CAD build for the part. Positions are in the model's coordinates, mm. Face numbers are marked on the shaded views. A direction names the side the tool comes from. Coordinates: 2 decimals unless noted, no trailing zeros. One line per item, written item: value.
from build123d import *

# Parameters (mm, degrees)
ESBO_O1_R           = 19
ESBO_O1_R_2         = 15
CONTRA_CENTRO_DEPTH = 12
CHANFRO1_SIZE       = 3.5
CHANFRO1_SIZE2      = 2


with BuildPart() as part:
    # Esboço1 → CONTRA CENTRO (new body)
    with BuildSketch(Plane.XY):
        Circle(ESBO_O1_R)
        Circle(ESBO_O1_R_2, mode=Mode.SUBTRACT)
    extrude(amount=CONTRA_CENTRO_DEPTH)

    # Chanfro1
    chanfro1_edges = [part.edges().sort_by_distance(p)[0] for p in [
        (-19, 0, 0),
    ]]
    chanfro1_side = [part.faces().sort_by_distance(p)[0] for p in [
        (-18.462598846, 0, 0),
    ]]
    chamfer(chanfro1_edges, length=CHANFRO1_SIZE, length2=CHANFRO1_SIZE2, reference=chanfro1_side[0])

    # Esboço2 → AA26234 (revolve)
    with BuildSketch(Plane(origin=(0, 0, 0), x_dir=(0, 0, -1), z_dir=(1, 0, 0)), mode=Mode.PRIVATE) as aa26234_sk:
        Polygon((-2.5, 19), (-10, 19), (-10, 24.5), (-12, 27.437165192), (-11.173430596, 28), (-9, 24.808137652), (-9, 20), (-7.5, 20), (-7.5, 23.763932023), (-9.894427191, 28.552786405), (-9, 29), (-6.5, 24), (-6.5, 20), (-5.5, 20), (-5.5, 23.763932023), (-7.894427191, 28.552786405), (-7, 29), (-4.5, 24), (-4.5, 20), (-3.5, 20), (-3.5, 23.763932023), (-5.894427191, 28.552786405), (-5, 29), (-2.5, 24), align=None)
    revolve(aa26234_sk.sketch.rotate(Axis((0, 0, 10), (0, 0, -1)), 90), axis=Axis((0, 0, 10), (0, 0, -1)))


solid = part.part
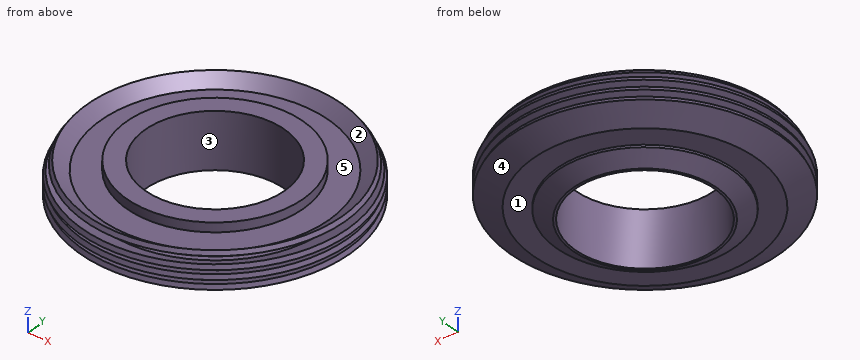
Q1. Mould opens along Z. For the marked faces 3, 4 and 5 say: released by +Z, released by -Z, zero draft, split by the parting line, or undercut.
Recorded:
face 3: zero draft
face 4: released by -Z
face 5: released by +Z
Q2. Drill centre lines: line 1 along Z through (x, y) = (-19, 8.5); line 2 along Z through (x, y) = (3, 24); line 3 along Y through (x, z) = (0, 4.75). Where is each one in solid material? Low to high.
Recorded:
line 1: z = 2.5 to 3.5, 4.5 to 5.5, 6.5 to 7.5, 9 to 10
line 2: z = 2.59 to 3.71, 4.59 to 5.71, 6.59 to 7.71, 9 to 10
line 3: y = -28.5 to -26.26, -24.5 to -15, 15 to 24.5, 26.26 to 28.5
Q3. Slice it at A-A (y = 22.5). Give the number of separate pieces and of enclosed holes in the cut face, plus the area to 3 significant figures.
Recorded:
separate pieces: 4
enclosed holes: 0
area: 150 mm^2
Q4. Which spindle directions (+Z, -Z, +X, -X, +Y, -Y) get a long thin tool onto all of the face, cutting with end or side? Do the marked faces 1 and 2. Say none if no direction does.
Recorded:
face 1: -Z
face 2: +Z
Q5. Pin check, flat tips, straight feed: pin 1 Ø6 at (y, z) = (-11.5, 1.5) entering from -X; pin 2 Ø1 at (x, y) = (-21.5, 14) entering from +Z; pin 3 Ø3 at (x, z) = (6.5, 9.5) entering from -Y; pin 4 Ø1 at (x, y) = (-13, -2) entering from -Z. Stop position of each tip, or through.
Recorded:
pin 1: stops at x = -25.66
pin 2: stops at z = 11.13
pin 3: stops at y = -28.55
pin 4: passes through
